Study the drawing (mm; zero at the part's minimum x, y, z) and answer. Round coordinates to 2 decimals unless told otherwise and drop trailing zeros. Write each loop counter-clockwise with the first axis right and the second up, starting at its lowest first coordinate (ties: lowest second). Pieces come first, ordered by that corner, then holes.
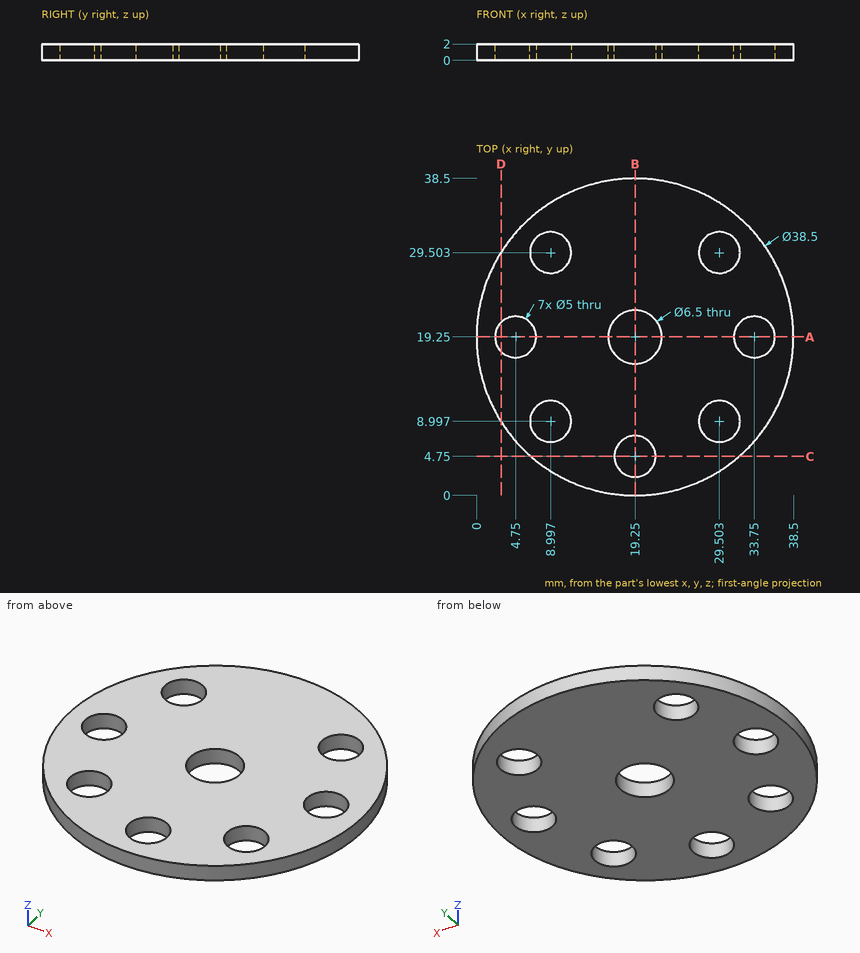
Q1. Find section A-A (y = 19.25). Determine the outline of the cut face in (x, z), plus the area to 3 significant figures.
Q2. Find section D-D (x = 3). Determine the outline of the cut face in (y, z), plus the area to 3 significant figures.
Q3. Find section B-B (x = 19.25). Determine the outline of the cut face in (y, z), plus the area to 3 significant figures.
Q4. Given pin 1 (1 mm diameter, centred on x = 4.5, z = 1.5, fed in from +Y); pin 2 (3 mm diameter, centred on x = 33, y = 15.5, fed in from -Z); pin 3 (1 mm diameter, centred on y = 17, z = 1, fed in from -X); pin 4 (3 mm diameter, centred on x = 33.75, y = 19.25, fed in from +Z), each flat-ended and moving along its own axis, determine where each tip first touches the part or whether it passes through.
Q5. Find section C-C (y = 4.75). Determine the outline of the cut face in (x, z).
Q6. Find the intervals of material crossed by L1, parallel to Y at x = 31, z = 0.5; L2, parallel to Y at x = 20, z = 1.85 (1 decimal); L3, parallel to Y at x = 35.5, z = 0.6 (1 decimal), in increasing order.
Report:
1. outline: (0, 0) - (2.25, 0) - (2.25, 2) - (0, 2) - close; (7.25, 0) - (16, 0) - (16, 2) - (7.25, 2) - close; (22.5, 0) - (31.25, 0) - (31.25, 2) - (22.5, 2) - close; (36.25, 0) - (38.5, 0) - (38.5, 2) - (36.25, 2) - close
1. area: 44.0 mm2
2. outline: (8.93, 0) - (17.46, 0) - (17.46, 2) - (8.93, 2) - close; (21.04, 0) - (29.57, 0) - (29.57, 2) - (21.04, 2) - close
2. area: 34.1 mm2
3. outline: (0, 0) - (2.25, 0) - (2.25, 2) - (0, 2) - close; (7.25, 0) - (16, 0) - (16, 2) - (7.25, 2) - close; (22.5, 0) - (38.5, 0) - (38.5, 2) - (22.5, 2) - close
3. area: 54.0 mm2
4. pin 1: stops at y = 32.19
4. pin 2: stops at z = 0
4. pin 3: stops at x = 0.08
4. pin 4: passes through
5. outline: (6.59, 0) - (16.75, 0) - (16.75, 2) - (6.59, 2) - close; (21.75, 0) - (31.91, 0) - (31.91, 2) - (21.75, 2) - close
6. L1: y = 4 to 6.99, 11 to 27.5, 31.51 to 34.5
6. L2: y = 0 to 2.4, 7.1 to 16.1, 22.4 to 38.5
6. L3: y = 8.9 to 17.5, 21 to 29.6
